from build123d import *

# Parameters (mm, degrees)
SKETCH1_W           = 140
SKETCH1_H           = 145
BOSS_EXTRUDE1_DEPTH = 5
SKETCH2_W           = 10
SKETCH2_H           = 5
CUT_EXTRUDE1_DEPTH  = 164.343962239
SKETCH3_R           = 1.5
CUT_EXTRUDE2_DEPTH  = 5
SKETCH4_R           = 1.5
CUT_EXTRUDE3_DEPTH  = 164.343962239
SKETCH5_R           = 1.75
SKETCH5_W           = 41
SKETCH5_H           = 20.5
CUT_EXTRUDE4_DEPTH  = 164.343962239
FILLET1_R           = 10


with BuildPart() as part:
    # Sketch1 → Boss-Extrude1 (new body)
    with BuildSketch(Plane.XY):
        with Locations((0, -75)):
            Rectangle(SKETCH1_W, SKETCH1_H)
    extrude(amount=-BOSS_EXTRUDE1_DEPTH)

    # Sketch2 → Cut-Extrude1 (cut, through all)
    with BuildSketch(Plane.XY):
        Polygon((43.894042166, -134.5), (43.894042166, -131.5), (38.894042166, -131.5), (38.894042166, -134.5), (36.394042166, -134.5), (36.394042166, -139.5), (38.894042166, -139.5), (38.894042166, -144.5), (43.894042166, -144.5), (43.894042166, -139.5), (46.394042166, -139.5), (46.394042166, -134.5), align=None)
        with Locations((21.394042166, -137)):
            Rectangle(SKETCH2_W, SKETCH2_H)
        with Locations((-21.394042166, -137)):
            Rectangle(SKETCH2_W, SKETCH2_H)
        Polygon((-46.394042166, -134.5), (-43.894042166, -134.5), (-43.894042166, -131.5), (-38.894042166, -131.5), (-38.894042166, -134.5), (-36.394042166, -134.5), (-36.394042166, -139.5), (-38.894042166, -139.5), (-38.894042166, -144.5), (-43.894042166, -144.5), (-43.894042166, -139.5), (-46.394042166, -139.5), align=None)
        Polygon((-43.894042166, -15.5), (-43.894042166, -18.5), (-38.894042166, -18.5), (-38.894042166, -15.5), (-36.394042166, -15.5), (-36.394042166, -10.5), (-38.894042166, -10.5), (-38.894042166, -5.5), (-43.894042166, -5.5), (-43.894042166, -10.5), (-46.394042166, -10.5), (-46.394042166, -15.5), align=None)
        with Locations((-21.394042166, -13)):
            Rectangle(SKETCH2_W, SKETCH2_H)
        with Locations((21.394042166, -13)):
            Rectangle(SKETCH2_W, SKETCH2_H)
        Polygon((46.394042166, -15.5), (43.894042166, -15.5), (43.894042166, -18.5), (38.894042166, -18.5), (38.894042166, -15.5), (36.394042166, -15.5), (36.394042166, -10.5), (38.894042166, -10.5), (38.894042166, -5.5), (43.894042166, -5.5), (43.894042166, -10.5), (46.394042166, -10.5), align=None)
    extrude(amount=-CUT_EXTRUDE1_DEPTH, mode=Mode.SUBTRACT)

    # Sketch3 → Cut-Extrude2 (cut)
    with BuildSketch(Plane.XY):
        with Locations((31.394042166, -137)):
            Circle(SKETCH3_R)
        with Locations(Location((-31.394042166, -137, 0), (0, 0, 180))):
            Circle(SKETCH3_R)
        with Locations(Location((31.394042166, -13, 0), (0, 0, 180))):
            Circle(SKETCH3_R)
        with Locations((-31.394042166, -13)):
            Circle(SKETCH3_R)
    extrude(amount=-CUT_EXTRUDE2_DEPTH, mode=Mode.SUBTRACT)

    # Sketch4 → Cut-Extrude3 (cut, through all)
    with BuildSketch(Plane.XY):
        with Locations((65, -124)):
            Circle(SKETCH4_R)
        with Locations((27, -124)):
            Circle(SKETCH4_R)
        with Locations(Location((27, -26, 0), (0, 0, 180))):
            Circle(SKETCH4_R)
        with Locations(Location((65, -26, 0), (0, 0, 180))):
            Circle(SKETCH4_R)
        with Locations((-27, -26)):
            Circle(SKETCH4_R)
        with Locations((-65, -26)):
            Circle(SKETCH4_R)
        with Locations(Location((-65, -124, 0), (0, 0, 180))):
            Circle(SKETCH4_R)
        with Locations(Location((-27, -124, 0), (0, 0, 180))):
            Circle(SKETCH4_R)
    extrude(amount=-CUT_EXTRUDE3_DEPTH, mode=Mode.SUBTRACT)

    # Sketch5 → Cut-Extrude4 (cut, through all)
    with BuildSketch(Plane.XY):
        with Locations((25, -80.1)):
            Circle(SKETCH5_R)
        with Locations(Location((25, -69.9, 0), (0, 0, 180))):
            Circle(SKETCH5_R)
        with Locations(Location((-25, -80.1, 0), (0, 0, 180))):
            Circle(SKETCH5_R)
        with Locations((-25, -69.9)):
            Circle(SKETCH5_R)
        with Locations((0, -75)):
            Rectangle(SKETCH5_W, SKETCH5_H)
    extrude(amount=-CUT_EXTRUDE4_DEPTH, mode=Mode.SUBTRACT)

    # Fillet1
    fillet1_edges = [part.edges().sort_by_distance(p)[0] for p in [
        (70, -147.5, -2.5),
        (-70, -147.5, -2.5),
        (-70, -2.5, -2.5),
        (70, -2.5, -2.5),
    ]]
    fillet(fillet1_edges, radius=FILLET1_R)


solid = part.part
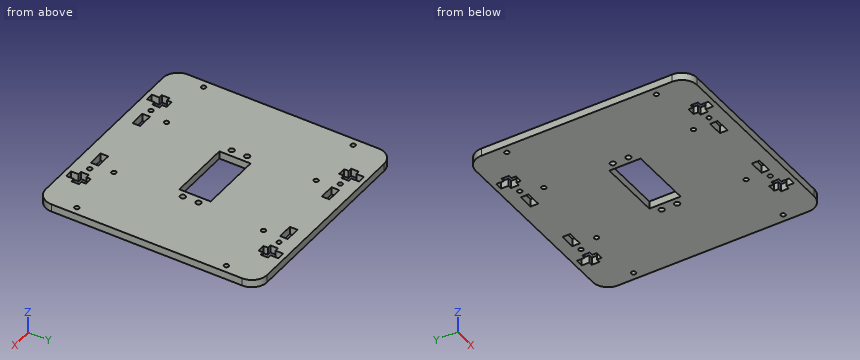
Could you check a few things on this model? Use its own coordinates, in mm. Coordinates: 2 decimals unless noted, no trailing zeros. Write each loop counter-clockwise with the first axis right and the second up, starting at its lowest first coordinate (ties: lowest second). Pieces come first, ordered by that corner, then holes. Notation, with made-up numbers: (17, -19.75) - (68, -19.75) arc R30 cw to (68, 15.25) - close; hole circle Ø8 at (49, 60.5). An arc over 180 degrees is marked (long way). Put each result on its own line as item: value. Start each with the question number.
Q1. I want a section at A-A on y = -69.9. Write out the boundary of the cut face in (x, z), plus the area to 3 significant figures.
Q2. I'm going to push flat-ended pins straight in: P1, Ø12, axis at x = -23, y = -60, coming from the +Z side; P2, Ø1.5, axis at y = -8, z = -1.5, coming from the +X side. Where does each tip first touch, or does it pass through?
Q3. I want a section at C-C on z = -4.2. Count the separate pieces of the cut face and the enclosed holes in it, plus the area to 3 significant figures.
Q4. I want a section at B-B on x = -41. Write out the boundary of the cut face in (y, z).
Q5. Please list where these lines run through material, in increasing order: L1, parallel to X at y = -124, z = -1.7; L2, parallel to Y at x = 25, z = -2; L3, parallel to Y at x = 44, z = -3.4.
Checks:
1. outline: (-70, -5) - (-26.75, -5) - (-26.75, 0) - (-70, 0) - close; (-23.25, -5) - (-20.5, -5) - (-20.5, 0) - (-23.25, 0) - close; (20.5, -5) - (23.25, -5) - (23.25, 0) - (20.5, 0) - close; (26.75, -5) - (70, -5) - (70, 0) - (26.75, 0) - close
1. area: 460 mm²
2. P1: z = 0
2. P2: x = 69.27
3. separate pieces: 1
3. enclosed holes: 25
3. area: 18,700 mm²
4. outline: (-147.5, -5) - (-144.5, -5) - (-144.5, 0) - (-147.5, 0) - close; (-131.5, -5) - (-18.5, -5) - (-18.5, 0) - (-131.5, 0) - close; (-5.5, -5) - (-2.5, -5) - (-2.5, 0) - (-5.5, 0) - close
5. L1: -70 to -66.5, -63.5 to -28.5, -25.5 to 25.5, 28.5 to 63.5, 66.5 to 70
5. L2: -147.5 to -139.5, -134.5 to -81.85, -78.35 to -71.65, -68.15 to -15.5, -10.5 to -2.5
5. L3: -147.5 to -139.5, -134.5 to -15.5, -10.5 to -2.5
